```python
from build123d import *

# Parameters (mm, degrees)
CYLINDER1033_W               = 6
CYLINDER1033_H               = 1.5
CYLINDER1033_ANGLE           = 180
CYLINDER1029_R               = 7.5
CYLINDER1029_DEPTH           = 5
CYLINDER1029_PITCH_ANGLE     = 90
THICKNESS001_T               = -1.5
BOX025_W                     = 4
BOX025_H                     = 1.5
BOX025_DEPTH                 = 12
CYLINDER1027_R               = 5
CYLINDER1027_DEPTH           = 40
CYLINDER1027_PITCH_ANGLE     = 90
CYLINDER1026_W               = 14
CYLINDER1026_H               = 10
CYLINDER1026_ANGLE           = 165
CYLINDER1026_ROLL_ANGLE      = 90
CYLINDER1026_PITCH_ANGLE     = 65
CYLINDER1026_PLACEMENT_ANGLE = 90
CONE001_ANGLE                = 165
CONE001_ROLL_ANGLE           = 90
CONE001_PITCH_ANGLE          = 65
CONE001_PLACEMENT_ANGLE      = 90


with BuildPart() as cylinder1047:
    # Cylinder1033 → Cylinder1033 (revolve)
    with BuildSketch(Plane(origin=(0, 70.75, 15), x_dir=(0, 0, 1), z_dir=(1, 0, 0))):
        with Locations((3, 0.75)):
            Rectangle(CYLINDER1033_W, CYLINDER1033_H)
    revolve(axis=Axis((0, 70.75, 15), (0, -1, 0)), revolution_arc=CYLINDER1033_ANGLE)


with BuildPart() as thickness001:
    # Cylinder1029 → Cylinder1029 (new body)
    with BuildSketch(Plane.XY):
        Circle(CYLINDER1029_R)
    extrude(amount=CYLINDER1029_DEPTH)


with BuildPart() as thickness001_1:
    # Cylinder1029 pitch: moved
    add(thickness001.part.rotate(Axis((0, 0, 0), (0, 1, 0)), CYLINDER1029_PITCH_ANGLE))


with BuildPart() as thickness001_2:
    # Cylinder1029 placement: moved
    add(thickness001_1.part.moved(Location((45, 70, 15))))

    # Thickness001
    thickness001_openings = [thickness001_2.faces().sort_by_distance(p)[0] for p in [
        (50, 70, 15),
    ]]
    offset(amount=THICKNESS001_T, openings=thickness001_openings)


with BuildPart() as fusion028:
    # Box025 → Box025 (new body)
    with BuildSketch(Plane(origin=(46, 69.25, 9), x_dir=(1, 0, 0), z_dir=(0, 0, 1))):
        with Locations((2, 0.75)):
            Rectangle(BOX025_W, BOX025_H)
    extrude(amount=BOX025_DEPTH)

    # Fusion028: union Thickness001
    add(thickness001_2.part)


with BuildPart() as cylinder1042:
    # Cylinder1027 → Cylinder1027 (new body)
    with BuildSketch(Plane.XY):
        Circle(CYLINDER1027_R)
    extrude(amount=CYLINDER1027_DEPTH)


with BuildPart() as cylinder1042_1:
    # Cylinder1027 pitch: moved
    add(cylinder1042.part.rotate(Axis((0, 0, 0), (0, 1, 0)), CYLINDER1027_PITCH_ANGLE))


with BuildPart() as cylinder1042_2:
    # Cylinder1027 placement: moved
    add(cylinder1042_1.part.moved(Location((5, 70, 15))))


with BuildPart() as cylinder1041:
    # Cylinder1026 → Cylinder1026 (revolve)
    with BuildSketch(Plane.XZ):
        with Locations((7, 5)):
            Rectangle(CYLINDER1026_W, CYLINDER1026_H)
    revolve(axis=Axis((0, 0, 0), (0, 0, 1)), revolution_arc=CYLINDER1026_ANGLE)


with BuildPart() as cylinder1041_1:
    # Cylinder1026 roll: moved
    add(cylinder1041.part.rotate(Axis((0, 0, 0), (1, 0, 0)), CYLINDER1026_ROLL_ANGLE))


with BuildPart() as cylinder1041_2:
    # Cylinder1026 pitch: moved
    add(cylinder1041_1.part.rotate(Axis((0, 0, 0), (0, 1, 0)), CYLINDER1026_PITCH_ANGLE))


with BuildPart() as cylinder1041_3:
    # Cylinder1026 placement: moved
    add(cylinder1041_2.part.moved(Location((20, 70, 15))).rotate(Axis((20, 70, 15), (0, 0, 1)), CYLINDER1026_PLACEMENT_ANGLE))


with BuildPart() as cone001:
    # Cone001 → Cone001 (revolve)
    with BuildSketch(Plane.XZ):
        Polygon((0, 0), (14, 14), (0, 14), align=None)
    revolve(axis=Axis((0, 0, 0), (0, 0, 1)), revolution_arc=CONE001_ANGLE)


with BuildPart() as cone001_1:
    # Cone001 roll: moved
    add(cone001.part.rotate(Axis((0, 0, 0), (1, 0, 0)), CONE001_ROLL_ANGLE))


with BuildPart() as cone001_2:
    # Cone001 pitch: moved
    add(cone001_1.part.rotate(Axis((0, 0, 0), (0, 1, 0)), CONE001_PITCH_ANGLE))


with BuildPart() as cone001_3:
    # Cone001 placement: moved
    add(cone001_2.part.moved(Location((6, 70, 15))).rotate(Axis((6, 70, 15), (0, 0, 1)), CONE001_PLACEMENT_ANGLE))


with BuildPart() as part_mirroring004:
    # Part__Mirroring004: instance of Cone001
    add(cone001_3.part.mirror(Plane(origin=(25, 0, 0), x_dir=(0, -1, 0), z_dir=(1, 0, 0))))


with BuildPart() as fusion050:
    # Part__Mirroring001: instance of Fusion028
    add(fusion028.part.mirror(Plane(origin=(25, 0, 0), x_dir=(0, -1, 0), z_dir=(1, 0, 0))))

    # Fusion031: union Fusion028, Cylinder1042, Cylinder1041, Part__Mirroring004, Cone001
    add(fusion028.part)
    add(cylinder1042_2.part)
    add(cylinder1041_3.part)
    add(part_mirroring004.part)
    add(cone001_3.part)

    # Fusion050: union Cylinder1047
    add(cylinder1047.part)


solid = fusion050.part
```
Could you check a few things on this model? Use its own coordinates, in mm. A direction names the side the tool comes from. Coordinates: 2 decimals unless noted, no trailing zeros. Order: outer loops, then holes, each group sorted by start corner. A loop starts at its lowest first (then second) coordinate and runs counter-clockwise, first axis right, second up. Notation, with made-up numbers: M -2.5,10.25 L 24.5,10.25 A18 ccw 24.5,40.25 Z; hole C 17,46 d8. An arc over 180 degrees is marked long. Use one line per item in the form item = value. Start each with the question number.
1. On a 3-axis mill with a long thin cutter (end or side, diameter ignored), from which of +Z, -Z, +X, -X, +Y, -Y can I reach the whole of each face in a straight line? I mean faces 1 (the flat face through (48, 70.75, 15)), 2 (the flat face through (3.5, 67, 15)), 3 (the cylindrical face through (24.72, 65.564, 12.693)). Say none if no direction works.
2. Suppose I cut it at C-C on x = 9.5. Write out the boundary of the cut face in (y, z).
3. Suppose I cut it at A-A on y = 70. Write out the boundary of the cut face in (x, z).
4. Suppose I cut it at B-B on x = 27. Write out the boundary of the cut face in (y, z), then the cut area to 3 significant figures.
5. For pin 1 (4 mm diameter, centred on x = 42.5, z = 13.5, fed in from +Y); pin 2 (6 mm diameter, centred on y = 67, z = 13, fed in from -X); pin 3 (2.5 mm diameter, centred on y = 73, z = 14, fed in from -X); pin 4 (3 mm diameter, centred on x = 1, z = 13.5, fed in from +Y), each with a flat end and sliding along its axis, tell me the tip position at first contact or that it passes through.
6. Please list where these lines run through material, in increasing order: line 1 (Y direction, x = 1, z = 12.25); line 2 (X direction, y = 64.5, z = 14.5); line 3 (X direction, y = 67.75, z = 8.75).
7. We'd pull the mould along Y, two halves only. Please class faces 4 (the flat face through (0, 76, 13)), 5 (the cylindrical face through (47.465, 65.436, 20.952)), 6 (the cylindrical face through (48, 64, 15)): +Y half, -Y half, draft (parallel to the pull), parting line (faces both ways), or undercut.
Geometry says:
q1.face_1 = +X
q1.face_2 = -X
q1.face_3 = none
q2.outline = C 70,15 d10
q3.outline = M 0,7.5 L 5,7.5 L 5,10 L 45,10 L 45,7.5 L 50,7.5 L 50,22.5 L 45,22.5 L 45,20 L 39,20 L 30,29 L 20,29 L 11,20 L 5,20 L 5,22.5 L 0,22.5 L 0,21 A6 ccw 0,9 Z
q4.outline = M 67.57,28.79 L 69.13,19.92 A5 ccw long 72.11,10.47 L 75.92,2.31 A14 ccw Z
q4.area = 325 mm^2
q5.pin_1 = 75
q5.pin_2 = -6
q5.pin_3 = 3.5
q5.pin_4 = 77.5
q6.line_1 = 63.02 to 64.67, 69.25 to 70.75, 75.33 to 76.98
q6.line_2 = 3.5 to 5, 45 to 46.5
q6.line_3 = 0 to 5, 45 to 50
q7.face_4 = draft
q7.face_5 = parting line
q7.face_6 = undercut
